The model under review builds one solid part; all positions refer to its coordinate system, in mm. Face numbers are marked on the shaded views. A direction names the side the tool comes from. Coordinates: 2 decimals unless noted, no trailing zeros. Loops run counter-clockwise (first coordinate to the right, second up) from the corner with the lowest first, then second, coordinate; pieces in that order, holes last. Notation, with made-up numbers: (47.25, 41.5) - (82.25, 41.5) arc R17 ccw to (82.25, 58.5) - close; hole circle Ø9 at (41.5, 0.25). An arc over 180 degrees is marked (long way). Answer in a Markdown table with one row per item. Add a question column.
(1) We need section B-B on z = 19. Write out the cut boundary in (x, y) (3 decimals).
(2) Machinability: for the marked faces 1 and 2, which of the approach directions +Z, -Z, +X, -X, +Y, -Y give a long, thin tool a straight path to every point of the face, cutting with its end or side? Answer none if there is none.
(3) For line 1 along X through (y, z) = (0, 104); line 2 along X through (y, z) = (0, 9); line 3 along Y through (x, z) = (64.5, 21.5), list the stretches that pass through material, from the lowest coordinate up.
(4) We need section A-A on z = 94.5. Write out the cut boundary in (x, y), plus the area to 3 significant figures.
(5) Mouldability with a two-part tool opening along X and no side actions: class the marked faces 3, 4 and 5 as +X half, -X half, draft (parallel to the pull), parting line (faces both ways), or undercut.
(6) For P1, Ø5, axis at y = -16.5, z = 64, coming from the -X side; P2, Ø1, axis at y = 2.5, z = 58, coming from the -X side; P3, Ø8, axis at x = 60, z = 46.5, coming from the +Y side, all flat-tipped, find the tip position at first contact; note any pin that passes through.
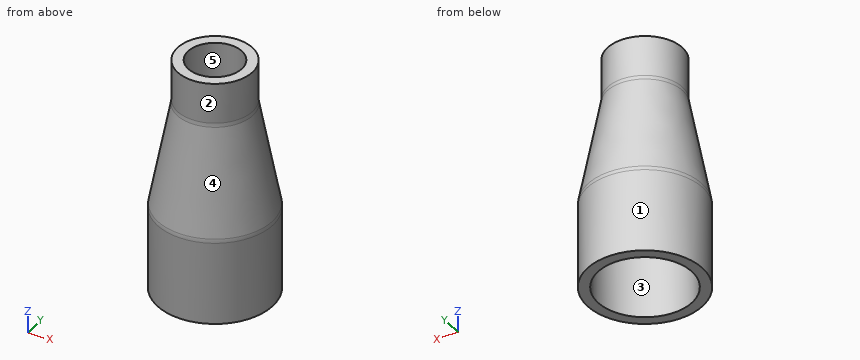
Autodesk Fusion 360 part; units mm, degrees
sketch "Sketch12" plane through (0, 0, 0) normal (0, 1, 0) x (1, 0, 0)
  line L0 (90.9618, -0.0199) -> (90.9618, -40.0199)
  line L1 (90.9618, -40.0199) -> (81.4368, -90.0199)
  line L2 (81.4368, -90.0199) -> (81.4368, -110.0199)
  line L3 (81.4368, -110.0199) -> (76.4368, -110.0199)
  line L4 (76.4368, -110.0199) -> (76.4368, -90.0199)
  line L5 (76.4368, -90.0199) -> (85.9618, -40.0199)
  line L6 (85.9618, -40.0199) -> (85.9618, -0.0199)
  line L7 (85.9618, -0.0199) -> (90.9618, -0.0199)
  line L8 (63.7368, -110.603) -> (63.7368, -0.0809)
  dimension "d16" = 5
  dimension "d17" = 5
  dimension "d18" = 50
  dimension "d19" = 20
  dimension "d20" = 40
  dimension "d21" = 12.7
  dimension "d27" = 22.225
revolve "Revolve1" add sketch "Sketch12" angle 360 about axis through (63.7368, 0, 110.603) along (0, 0, -1)
fillet "Fillet1" radius 10 1 edges at (47.2346, -6.4006, 90.0199)
fillet "Fillet2" radius 10 1 edges at (38.3542, -9.845, 40.0199)
Outcome:
| question | item | result |
|---|---|---|
| 1 | outline | circle Ø54.45 at (63.737, 0); hole circle Ø44.45 at (63.737, 0) |
| 2 | face 1 | +Z, -Z |
| 2 | face 2 | +Z |
| 3 | line 1 | 46.04 to 51.04, 76.44 to 81.44 |
| 3 | line 2 | 36.51 to 41.51, 85.96 to 90.96 |
| 3 | line 3 | -27.21 to -22.21, 22.21 to 27.21 |
| 4 | outline | circle Ø35.4 at (63.74, 0); hole circle Ø25.4 at (63.74, 0) |
| 4 | area | 478 mm² |
| 5 | face 3 | undercut |
| 5 | face 4 | parting line |
| 5 | face 5 | undercut |
| 6 | P1 | x = 45.83 |
| 6 | P2 | x = 39.96 |
| 6 | P3 | y = 26.6 |
